Check sheet for the drawn part. Datum: minimum x, y, z corner. Units: mm. A direction names the side the tool comes from. Round coordinates to 2 decimals unless told otherwise and drop trailing zeros. Write each loop counter-clockwise with the first axis right and the second up, starting at its lowest first coordinate (ties: lowest second). Pieces come first, ordered by that corner, then holes. Notation, with made-up numbers: (67, 21) - (79, 21) arc R10 ccw to (79, 26) - close; hole circle Ø1 at (-14.5, -28.5). An arc over 180 degrees is marked (long way). Answer as a JSON object with one key per item and string values. Group by question number.
Item 1: Sectioned sample at D-D on z = 23.5. Record the boundary of the cut face in (x, y) (1 decimal).
Item 2: Thickness scan on line 1 (X direction, y = 0.2, z = 39.37); line 2 (Z direction, x = 15.24, y = 0.45); line 3 (X direction, y = 0.4, z = 4). Record the ranges inside material, lowest first.
Item 3: Gauge pin test, flat ends, axial feed: P1, Ø2.5, axis at x = 27, z = 38, coming from the +Y side; P2, Ø3, axis at x = 33.5, z = 37, coming from the +Y side; P3, Ø1, axis at x = 27, y = 1.5, coming from the -Z side. Record the tip position at first contact, or that the pin passes through.
Item 4: Sectioned sample at B-B on x = 3.81. Record the boundary of the cut face in (y, z) (1 decimal), plus the area to 3 significant figures.
Item 5: Set-up check for the marked faces 1 and 2: record each of +Z, -Z, +X, -X, +Y, -Y from which the full face is reachable in a straight line by a thin tool's end or side.
Item 6: Sectioned sample at C-C on z = 3.81. Record the boundary of the cut face in (x, y) (1 decimal).
Item 7: Sectioned sample at A-A on x = 36.83. Record the boundary of the cut face in (y, z) (1 decimal).
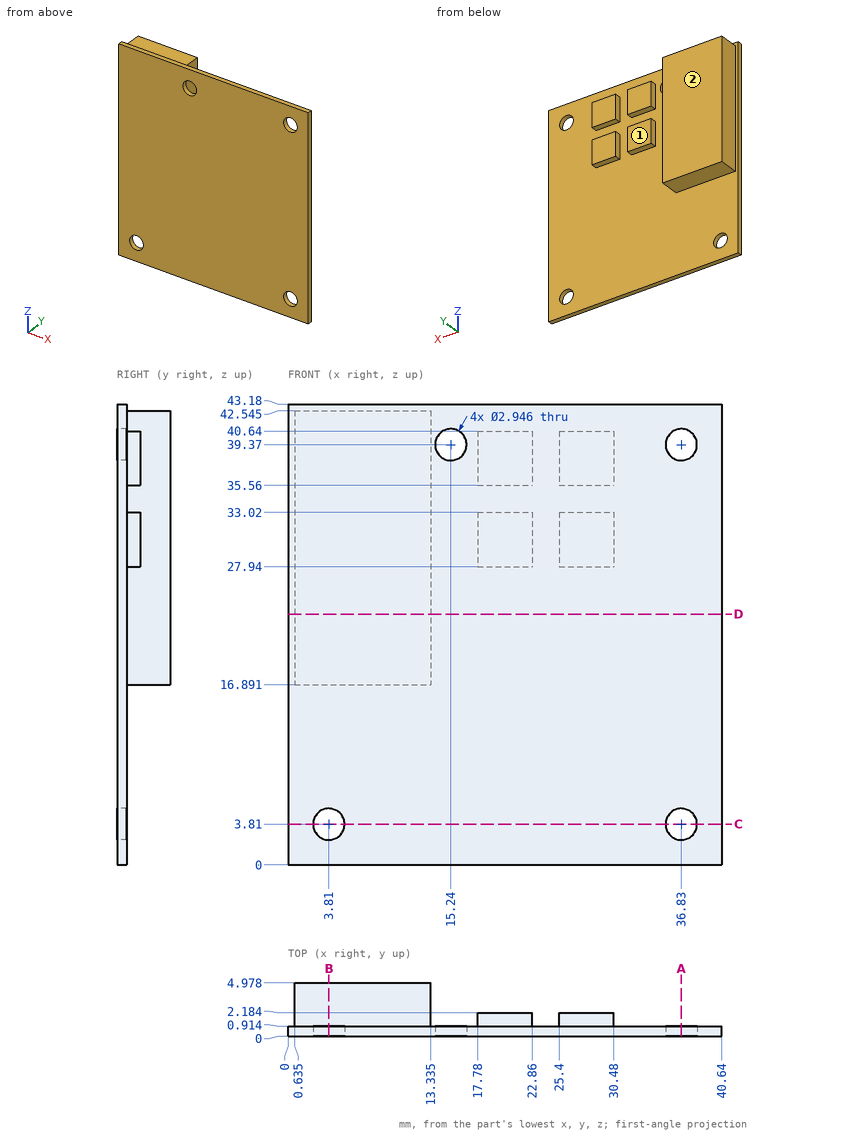
Completed:
{
 "1": {"outline": "(0, 0) - (40.6, 0) - (40.6, 0.9) - (13.3, 0.9) - (13.3, 5) - (0.6, 5) - (0.6, 0.9) - (0, 0.9) - close"},
 "2": {"line 1": "0 to 13.77, 16.71 to 35.36, 38.3 to 40.64", "line 2": "0 to 37.9, 40.84 to 43.18", "line 3": "0 to 2.35, 5.27 to 35.37, 38.29 to 40.64"},
 "3": {"P1": "y = 2.18", "P2": "y = 0.91", "P3": "z = 27.94"},
 "4": {"outline": "(0, 0) - (0.9, 0) - (0.9, 2.3) - (0, 2.3) - close; (0, 5.3) - (0.9, 5.3) - (0.9, 16.9) - (5, 16.9) - (5, 42.5) - (0.9, 42.5) - (0.9, 43.2) - (0, 43.2) - close", "area": "141 mm²"},
 "5": {"face 1": "+Z, -Z, +X, +Y", "face 2": "+Z, -Z, +X, -X, +Y"},
 "6": {"outline": "(0, 0) - (2.3, 0) - (2.3, 0.9) - (0, 0.9) - close; (5.3, 0) - (35.4, 0) - (35.4, 0.9) - (5.3, 0.9) - close; (38.3, 0) - (40.6, 0) - (40.6, 0.9) - (38.3, 0.9) - close"},
 "7": {"outline": "(0, 0) - (0.9, 0) - (0.9, 2.3) - (0, 2.3) - close; (0, 5.3) - (0.9, 5.3) - (0.9, 37.9) - (0, 37.9) - close; (0, 40.8) - (0.9, 40.8) - (0.9, 43.2) - (0, 43.2) - close"}
}
